from build123d import *

# Parameters (mm, degrees)
ESBO_O1_W                = 20
ESBO_O1_H                = 20
ESBO_O1_R                = 3
RESSALTO_EXTRUS_O1_DEPTH = 86
ESBO_O2_W                = 8
ESBO_O2_H                = 1.75
CORTE_EXTRUS_O1_DEPTH    = 173.580416038
PADR_OCIRCULAR2_COUNT    = 4
FILETE2_R                = 1
FILETE3_R                = 2
FILETE4_R                = 0.25


with BuildPart() as part:
    # Esboço1 → Ressalto-extrusão1 (new, symmetric)
    with BuildSketch(Plane(origin=(0, 0, 0), x_dir=(1, 0, 0), z_dir=(0, 1, 0))):
        Rectangle(ESBO_O1_W, ESBO_O1_H)
        with Locations(Location((0, 0, 0), (0, 0, 270))):
            Circle(ESBO_O1_R, mode=Mode.SUBTRACT)
    extrude(amount=RESSALTO_EXTRUS_O1_DEPTH, both=True)

    # Esboço2 → Corte-extrusão1 (cut, through all)
    with BuildSketch(Plane(origin=(0, 86, 0), x_dir=(1, 0, 0), z_dir=(0, 1, 0))):
        Polygon((-7.05, 8.25), (-2.8, 4), (2.8, 4), (7.05, 8.25), (4, 8.25), (-4, 8.25), align=None)
        with Locations((0, 9.125)):
            Rectangle(ESBO_O2_W, ESBO_O2_H)
    corte_extrus_o1 = extrude(amount=-CORTE_EXTRUS_O1_DEPTH, mode=Mode.SUBTRACT)

    # PadrãoCircular2: Corte-extrusão1 ×4 about axis
    padr_ocircular2_axis = Axis((0, 0, 0), (0, 1, 0))
    for i in range(1, PADR_OCIRCULAR2_COUNT):
        add(corte_extrus_o1.rotate(padr_ocircular2_axis, i * 360 / PADR_OCIRCULAR2_COUNT), mode=Mode.SUBTRACT)

    # Filete2
    filete2_edges = [part.edges().sort_by_distance(p)[0] for p in [
        (10, 0, 10),
        (-10, 0, 10),
        (-10, 0, -10),
        (10, 0, -10),
    ]]
    fillet(filete2_edges, radius=FILETE2_R)

    # Filete3
    filete3_edges = [part.edges().sort_by_distance(p)[0] for p in [
        (-4, 0, 2.8),
        (2.8, 0, -4),
        (-2.8, 0, -4),
        (2.8, 0, 4),
    ]]
    fillet(filete3_edges, radius=FILETE3_R)

    # Filete4
    filete4_edges = [part.edges().sort_by_distance(p)[0] for p in [
        (-8.25, 0, -7.05),
        (-8.25, 0, 7.05),
        (7.05, 0, -8.25),
        (-7.05, 0, -8.25),
        (8.25, 0, 7.05),
        (8.25, 0, -7.05),
        (-7.05, 0, 8.25),
        (7.05, 0, 8.25),
    ]]
    fillet(filete4_edges, radius=FILETE4_R)


solid = part.part
Source: CAD feature listing. Evaluate the final solid. Frame: model axes, mm. A direction names the side the tool comes from. Coordinates: 2 decimals unless noted, no trailing zeros. Loops run counter-clockwise (first coordinate to the right, second up) from the corner with the lowest first, then second, coordinate; pieces in that order, holes last. Notation, with made-up numbers: M 37.25,76 L 92.25,76 A19 cw 92.25,84 Z; hole C 3,28 d3. An arc over 180 degrees is marked long. Answer in a Markdown table with one row per item.
Q1. Section A-A on x = 0. Return the cut outline in (y, z).
Answers below:
| item | result |
|---|---|
| outline | M -86,-4 L 86,-4 L 86,-3 L -86,-3 Z; M -86,3 L 86,3 L 86,4 L -86,4 Z |
Q2. Set-up query: faces 1 (the flat face through (0, 1, -4)), 2 (the flat face through (5.9, 1.2, 4.7)), 3 (the flat face through (-4, 1, 0)), 4 (the flat face through (0, 1, 4)). Return all of +Z, -Z, +X, -X, +Y, -Y with unobstructed straight access to the full face (end or side cutting, diameter ignored); none if empty.
Answers below:
| item | result |
|---|---|
| face 1 | -Z, +Y, -Y |
| face 2 | +Y, -Y |
| face 3 | -X, +Y, -Y |
| face 4 | +Z, +Y, -Y |
Q3. Draft query along Z for faces 5 (the flat face through (6, 1, -10)), 6 (the flat face through (5, 1.2, -6.2)), 7 (the flat face through (-10, 1, -6)), 8 (the flat face through (-7, 1, 10)). Return one class per face: pulls with the +Z half, pulls with the -Z half, needs draft (parallel to the pull), parting line crosses it, or undercut.
Answers below:
| item | result |
|---|---|
| face 5 | pulls with the -Z half |
| face 6 | undercut |
| face 7 | needs draft |
| face 8 | pulls with the +Z half |
Q4. Section B-B on z = 0. Return the cut outline in (x, y).
Answers below:
| item | result |
|---|---|
| outline | M -4,-86 L -3,-86 L -3,86 L -4,86 Z; M 3,-86 L 4,-86 L 4,86 L 3,86 Z |
Q5. Ray query, probe 1 along X at (y, z) = (-2, 8.5); probe 2 along Z at (x, y) = (8, 38); probe 3 along X at (y, z) = (36, 0). Return the intervals inside material, ascending. Write a range as from..to.
Answers below:
| item | result |
|---|---|
| probe 1 | x = -10..-4, 4..10 |
| probe 2 | z = -10..-6.7, 6.7..10 |
| probe 3 | x = -4..-3, 3..4 |
Q6. First-contact query: pin 1 (8 mm diameter, centred on x = 5.5, z = 7, fed in from +Y); pin 2 (4 mm diameter, centred on y = 42, z = 0.5, fed in from -X); pin 3 (1.2 mm diameter, centred on x = -0.5, y = 24.5, fed in from -Z). Flat tips, straight axial feed; report the tip coordinate or a pass-through.
Answers below:
| item | result |
|---|---|
| pin 1 | stops at y = 86 |
| pin 2 | stops at x = -4.07 |
| pin 3 | stops at z = -4 |
